The drawing under review shows one solid part. Ordinate dimensions are in mm from its lowest x, y, z. A direction names the side the tool comes from. Give positions to 0.01 mm unless a question says otherwise; leave off trailing zeros. Write each loop counter-clockwise with the first axis right and the second up, starting at its lowest first coordinate (ties: lowest second). Pieces come first, ordered by that corner, then holes. Notation, with made-up numbers: (65.25, 74) -> (85.25, 74) arc R20 cw to (85.25, 100) -> close; hole circle Ø6 at (37, 35.5). An arc over 180 degrees is marked (long way). Answer as a JSON object with one key per item and string values.
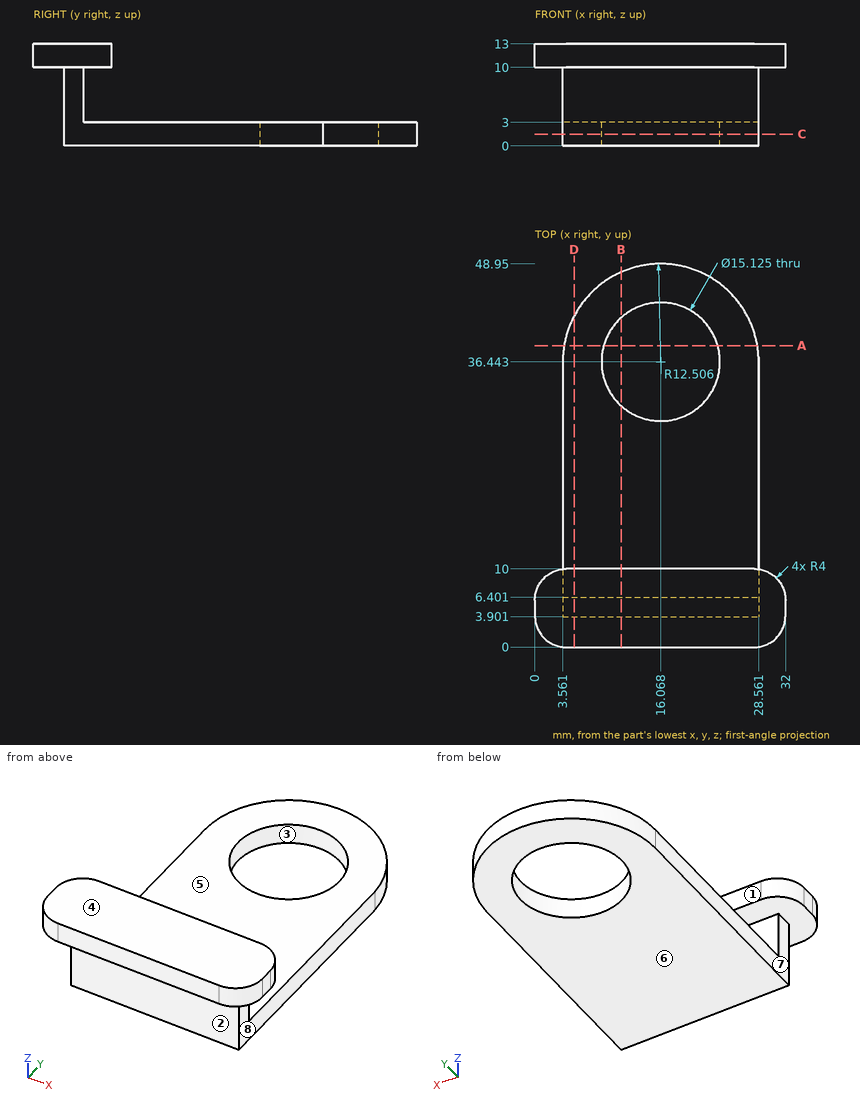
(1) The part is to be moulded in two halves that separate along Y. For the marked faces 1, 2, 3 and 4, say which applies: +Y half, -Y half, draft (parallel to the pull), parting line (faces both ways), or undercut.
Here are the results:
{"face 1": "+Y half", "face 2": "-Y half", "face 3": "undercut", "face 4": "draft"}
(2) We need section A-A, the plane y = 38.5. State the section outline as (x, z) points (1 decimal).
Here are the results:
{"outline": "(3.7, 0) -> (8.8, 0) -> (8.8, 3) -> (3.7, 3) -> close; (23.3, 0) -> (28.4, 0) -> (28.4, 3) -> (23.3, 3) -> close"}
(3) We need section B-B, the plane x = 11. State the section outline as (y, z) points.
Here are the results:
{"outline": "(0, 10) -> (3.9, 10) -> (3.9, 0) -> (30.83, 0) -> (30.83, 3) -> (6.4, 3) -> (6.4, 10) -> (10, 10) -> (10, 13) -> (0, 13) -> close; (42.06, 0) -> (47.88, 0) -> (47.88, 3) -> (42.06, 3) -> close"}
(4) For line 1 along Z through (x, y) = (25, 6.5); line 2 along Z through (x, y) = (20, 46.5); line 3 along Y through (x, z) = (27.5, 9), list the stretches that pass through material, from the lowest coordinate up.
Here are the results:
{"line 1": "z = 0 to 3, 10 to 13", "line 2": "z = 0 to 3", "line 3": "y = 3.9 to 6.4"}
(5) We need section C-C, the plane z = 1.5. State the section outline as (x, y) points (1 decimal).
Here are the results:
{"outline": "(3.6, 3.9) -> (28.6, 3.9) -> (28.6, 37) arc R12.5 ccw to (3.6, 36.4) -> close; hole circle Ø15.1 at (16.1, 36.4)"}
(6) We need section D-D, the plane x = 5. State the section outline as (y, z) points.
Here are the results:
{"outline": "(0, 10) -> (3.9, 10) -> (3.9, 0) -> (42.27, 0) -> (42.27, 3) -> (6.4, 3) -> (6.4, 10) -> (10, 10) -> (10, 13) -> (0, 13) -> close"}
(7) For the marked faces 5, 6, 7 and 8, list the 3-axis set-ups (+Z, -Z, +X, -X, +Y, -Y) from which the entire face can be reached by the end or side of a thin tool; tool diameter is ignored.
Here are the results:
{"face 5": "+X, -X, +Y", "face 6": "-Z, +X, -X, +Y, -Y", "face 7": "-Z, -X, +Y, -Y", "face 8": "-Z, +X, +Y, -Y"}
(8) Clearance check with flat-ended pins moving along their axes: pin 1 (12 mm diameter, centred on x = 16.5, y = 11, fed in from -Z); pin 2 (4 mm diameter, centred on x = 18.5, y = 27, fed in from +Z); pin 3 (1.5 mm diameter, centred on x = 16, z = 12, fed in from +Y); pin 4 (5 mm diameter, centred on y = 21.5, z = 1.5, fed in from +X). State where each tip first meets the part, or that it passes through.
Here are the results:
{"pin 1": "stops at z = 0", "pin 2": "stops at z = 3", "pin 3": "stops at y = 10", "pin 4": "stops at x = 28.56"}
